```python
from build123d import *

# Parameters (mm, degrees)
ESBO_O1_W                = 500
ESBO_O1_H                = 25
ESBO_O2_R                = 6
RESSALTO_EXTRUS_O1_DEPTH = 5


with BuildPart() as part:
    # Esboço1 → Revolução1 (revolve)
    with BuildSketch(Plane.XY):
        with Locations((0, 12.5)):
            Rectangle(ESBO_O1_W, ESBO_O1_H)
    revolve(axis=Axis((0, 0, 0), (1, 0, 0)))

    # Esboço2 → Ressalto-extrusão1 (add, symmetric)
    with BuildSketch(Plane.XY):
        with BuildLine():
            Line((250, -20), (250, 20))
            Line((250, 20), (285, 20))
            ThreePointArc((285, 20), (295.606601718, 15.606601718), (300, 5))
            Line((300, 5), (300, -5))
            ThreePointArc((300, -5), (295.606601718, -15.606601718), (285, -20))
            Line((285, -20), (250, -20))
        make_face()
        with Locations((290, 0)):
            Circle(ESBO_O2_R, mode=Mode.SUBTRACT)
    ressalto_extrus_o1 = extrude(amount=RESSALTO_EXTRUS_O1_DEPTH, both=True)

    # Espelhar1: Ressalto-extrusão1 across plane
    add(ressalto_extrus_o1.mirror(Plane(origin=(0, 0, 0), x_dir=(0, 0, 1), z_dir=(1, 0, 0))))


solid = part.part
```
Verification items for the finished model (mm, model axes). A direction names the side the tool comes from. Give positions to 0.01 mm unless a question says otherwise; leave off trailing zeros. Order: outer loops, then holes, each group sorted by start corner. A loop starts at its lowest first (then second) coordinate and runs counter-clockwise, first axis right, second up. Notation, with made-up numbers: M 10.25,81.5 L 62.25,81.5 A27 cw 62.25,110.5 Z; hole C 46.25,-19 d2. An arc over 180 degrees is marked long. Return JSON: item names as keys, results as strings. Group by question number.
1) Section check B-B on z = 0. Record the cut outline in (x, y), and give its area (3 significant figures).
2) Access from +Z, -Z, +X, -X, +Y, -Y to the whole of each face (thin tool, end or side, straight path). Record for faces 1 (the face through (275, 0, 5)), 2 (the face through (-275, 0, 5)), 3 (the face through (-275, 0, -5)), 4 (the face through (-268, -20, 0)).
3) Mould release check, pull along X, two halves, no side actions. Record for faces 5 (the face through (-295.723, 1.802, -0.07)), 6 (the face through (3.5, 23.846, 7.509)), 7 (the face through (295.72, -15.49, 0.07)), 8 (the face through (-295.49, 15.72, 0.07)): pulls with the +X half, pulls with the -X half, needs draft (parallel to the pull), parting line crosses it, or undercut.
4) Section check D-D on x = -116. Record the cut outline in (y, z), and give its area (3 significant figures).
5) Scan lines: line 1 (X direction, y = -0.5, z = -2.5); line 2 (X direction, y = 3, z = 3); line 3 (X direction, y = -15, z = -11). Record each from-to range of solid material in increasing order.
6) Go/stop test with flat-tipped pins: pin 1 Ø8 at (y, z) = (-15.5, -3.5) entering from -X; pin 2 Ø8 at (x, z) = (-272, -2) entering from +Y; pin 3 Ø12 at (x, y) = (30, -10) entering from -Z. Record where each tip stops, or that it passes through.
7) Section check A-A on y = 0. Record the cut outline in (x, z).
8) Section check C-C on x = -290. Record the cut outline in (y, z), and give its area (3 significant figures).
Answer block:
{
 "1": {"outline": "M -300,-5 A15 ccw -285,-20 L -250,-20 L -250,-25 L 250,-25 L 250,-20 L 285,-20 A15 ccw 300,-5 L 300,5 A15 ccw 285,20 L 250,20 L 250,25 L -250,25 L -250,20 L -285,20 A15 ccw -300,5 Z; hole C -290,0 d12; hole C 290,0 d12", "area": "28,600 mm^2"},
 "2": {"face 1": "+Z, +X, +Y, -Y", "face 2": "+Z, -X, +Y, -Y", "face 3": "-Z, -X, +Y, -Y", "face 4": "+Z, -Z, -X, -Y"},
 "3": {"face 5": "undercut", "face 6": "needs draft", "face 7": "pulls with the +X half", "face 8": "pulls with the -X half"},
 "4": {"outline": "C 0,0 d50", "area": "1,960 mm^2"},
 "5": {"line 1": "x = -300 to -295.98, -284.02 to 284.02, 295.98 to 300", "line 2": "x = -300 to -295.2, -284.8 to 284.8, 295.2 to 300", "line 3": "x = -250 to 250"},
 "6": {"pin 1": "stops at x = -298.52", "pin 2": "stops at y = 20", "pin 3": "stops at z = -24.68"},
 "7": {"outline": "M -300,-5 L -296,-5 L -296,5 L -300,5 Z; M -284,-5 L -250,-5 L -250,-25 L 250,-25 L 250,-5 L 284,-5 L 284,5 L 250,5 L 250,25 L -250,25 L -250,5 L -284,5 Z; M 296,-5 L 300,-5 L 300,5 L 296,5 Z"},
 "8": {"outline": "M -19.14,-5 L -6,-5 L -6,5 L -19.14,5 Z; M 6,-5 L 19.14,-5 L 19.14,5 L 6,5 Z", "area": "263 mm^2"}
}
